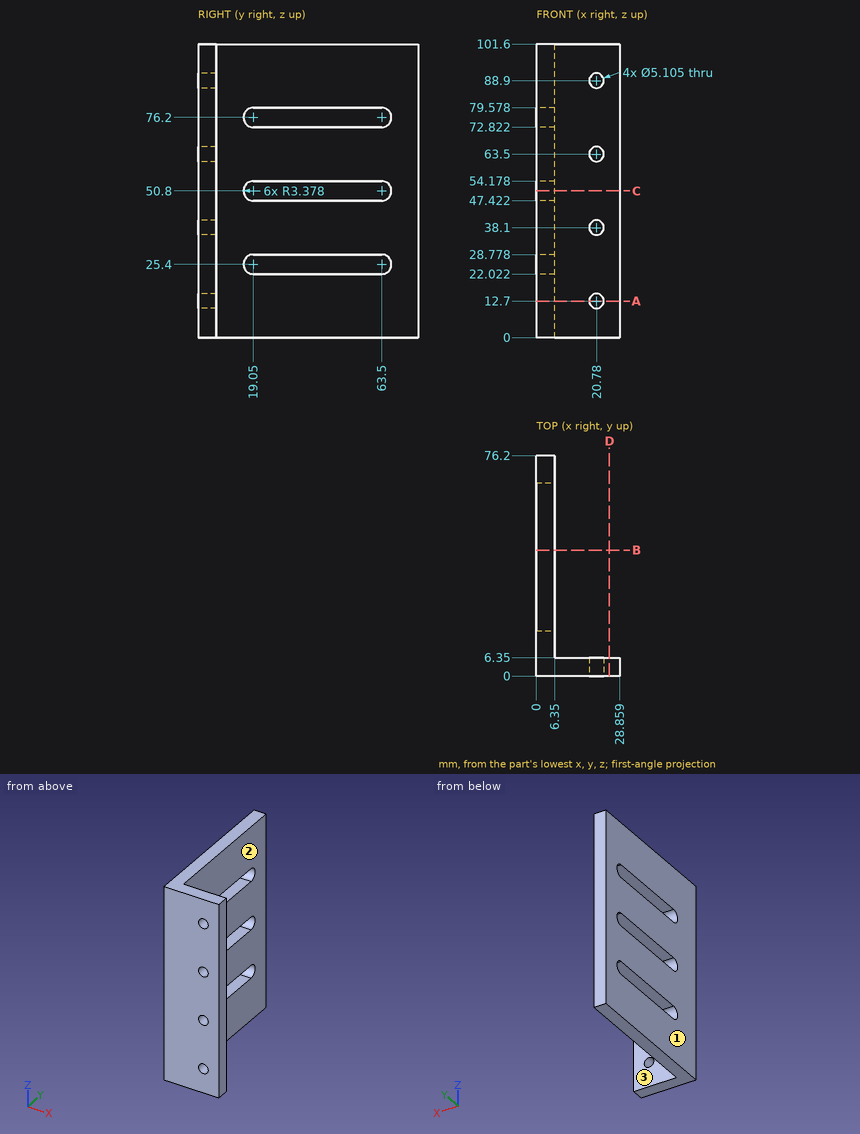
The drawing under review shows one solid part. Ordinate dimensions are in mm from its lowest x, y, z. Give positions to 0.01 mm unless a question says otherwise; leave off trailing zeros. Order: outer loops, then holes, each group sorted by start corner. A loop starts at its lowest first (then second) coordinate and runs counter-clockwise, first axis right, second up. Notation, with made-up numbers: (79.25, 1) -> (105.25, 1) arc R18 cw to (105.25, 5) -> close; hole circle Ø4 at (84.5, -19). An arc over 180 degrees is marked (long way). Write item = value, one per line. Start each with the question number.
(1) We need section A-A on z = 12.7. Write out the cut boundary in (x, y).
(2) For pin 1 (8 mm diameter, centred on x = 20.78, z = 12.7, fed in from +Y); pin 2 (2 mm diameter, centred on y = 55.5, z = 89.5, fed in from +X); pin 3 (4.5 mm diameter, centred on x = 20.78, z = 88.9, fed in from +Y) (3 decimals), all flat-tipped, find the tip position at first contact; note any pin that passes through.
(3) Mouldability with a two-part tool opening along X and no side actions: class the marked faces 1, 2 and 3 as +X half, -X half, draft (parallel to the pull), parting line (faces both ways), or undercut.
(4) We need section B-B on y = 43.5. Write out the cut boundary in (x, z).
(5) To check wall thickness, follow line 1 along Z through (x, y) = (4.75, 33); line 2 along X through (y, z) = (3, 88.9); line 3 along X through (y, z) = (19, 61.5). State the ranges of each line that lie inside material, in increasing order.
(6) We need section D-D on x = 25.25. Write out the cut boundary in (y, z), plus the area to 3 significant figures.
(7) We need section C-C on z = 50.8. Write out the cut boundary in (x, y).
Numbers:
q1.outline = (0, 0) -> (18.23, 0) -> (18.23, 6.35) -> (6.35, 6.35) -> (6.35, 76.2) -> (0, 76.2) -> close; (23.33, 0) -> (28.86, 0) -> (28.86, 6.35) -> (23.33, 6.35) -> close
q2.pin_1 = 6.35
q2.pin_2 = 6.35
q2.pin_3 = through
q3.face_1 = -X half
q3.face_2 = +X half
q3.face_3 = draft
q4.outline = (0, 0) -> (6.35, 0) -> (6.35, 22.02) -> (0, 22.02) -> close; (0, 28.78) -> (6.35, 28.78) -> (6.35, 47.42) -> (0, 47.42) -> close; (0, 54.18) -> (6.35, 54.18) -> (6.35, 72.82) -> (0, 72.82) -> close; (0, 79.58) -> (6.35, 79.58) -> (6.35, 101.6) -> (0, 101.6) -> close
q5.line_1 = 0 to 22.02, 28.78 to 47.42, 54.18 to 72.82, 79.58 to 101.6
q5.line_2 = 0 to 18.23, 23.33 to 28.86
q5.line_3 = 0 to 6.35
q6.outline = (0, 0) -> (6.35, 0) -> (6.35, 101.6) -> (0, 101.6) -> close
q6.area = 645 mm^2
q7.outline = (0, 0) -> (28.86, 0) -> (28.86, 6.35) -> (6.35, 6.35) -> (6.35, 15.67) -> (0, 15.67) -> close; (0, 66.88) -> (6.35, 66.88) -> (6.35, 76.2) -> (0, 76.2) -> close
